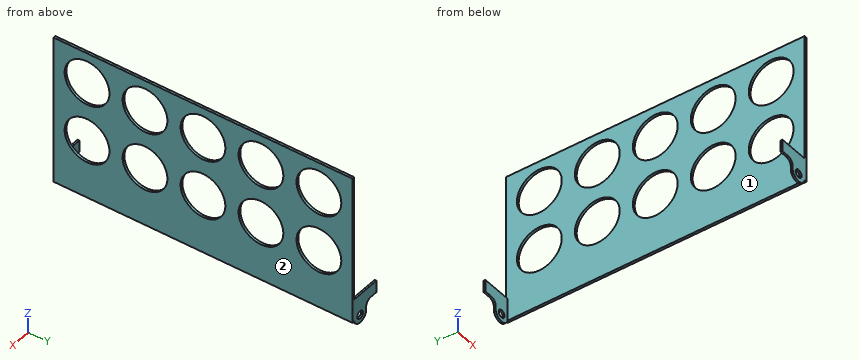
from build123d import *

# Parameters (mm, degrees)
F0_R     = 6.5
F1_DEPTH = 250
F2_W     = 494
F2_H     = 100
F3_DEPTH = 100
F4_R     = 10
F5_W     = 500
F5_H     = 250
F6_DEPTH = 4
F7_R     = 37.5
F8_DEPTH = 25


with BuildPart() as f1:
    # F0 (on Front) → F1 (new body, symmetric)
    with BuildSketch(Plane.XZ):
        with BuildLine():
            Line((-13.5, 15), (-13.5, 0))
            ThreePointArc((-13.5, 0), (-1.356871, -13.431638), (13.227245, -2.7))
            Line((13.227245, -2.7), (13.5, -2.7))
            Line((13.5, -2.7), (13.5, 15))
            Line((13.5, 15), (13.5, 35))
            Line((13.5, 35), (-36.5, 35))
            Line((-36.5, 35), (-36.5, 15))
            Line((-36.5, 15), (-13.5, 15))
        make_face()
        Circle(F0_R, mode=Mode.SUBTRACT)
    extrude(amount=F1_DEPTH, both=True)

    # F2 (on face) → F3 (cut)
    with BuildSketch(Plane.YZ.offset(13.5)):
        Rectangle(F2_W, F2_H)
    extrude(amount=-F3_DEPTH, mode=Mode.SUBTRACT)

    # F4
    f4_edges = [f1.edges().sort_by_distance(p)[0] for p in [
        (-13.5, 248.5, 15),
        (-13.5, -248.5, 15),
    ]]
    fillet(f4_edges, radius=F4_R)

    # F5 (on face) → F6 (join)
    with BuildSketch(Plane.YZ.offset(13.5)):
        with Locations((0, 122.3)):
            Rectangle(F5_W, F5_H)
    extrude(amount=F6_DEPTH)

    # F7 (on face) → F8 (cut)
    with BuildSketch(Plane.YZ.offset(17.5)):
        with Locations((-194, 95.8)):
            Circle(F7_R)
        with Locations((-194, 195.8)):
            Circle(F7_R)
        with Locations((-97, 95.8)):
            Circle(F7_R)
        with Locations((-97, 195.8)):
            Circle(F7_R)
        with Locations((0, 95.8)):
            Circle(F7_R)
        with Locations((0, 195.8)):
            Circle(F7_R)
        with Locations((97, 95.8)):
            Circle(F7_R)
        with Locations((97, 195.8)):
            Circle(F7_R)
        with Locations((194, 95.8)):
            Circle(F7_R)
        with Locations((194, 195.8)):
            Circle(F7_R)
    extrude(amount=-F8_DEPTH, mode=Mode.SUBTRACT)


solid = f1.part
Could you check a few things on this model? Use its own coordinates, in mm. Face numbers are marked on the shaded views. Coordinates: 2 decimals unless noted, no trailing zeros. Loops run counter-clockwise (first coordinate to the right, second up) from the corner with the lowest first, then second, coordinate; pieces in that order, holes last.
1. For P1, Ø3, axis at y = 78, z = 160.5, coming from the -X side; P2, Ø1.5, axis at x = -22.5, y = -248.5, coming from the +Z side; P3, Ø0.9, axis at y = -248.5, z = 1.5, coming from the -X side; P4, Ø21, axis at x = 0, z = 0, coming from the -Y side, each with a flat end and sliding along its axis, tell me the tip position at first contact or that it passes through.
2. We'd pull the mould along Y, two halves only. Please class the marked faces 1 and 2: released by +Y, released by -Y, zero draft, split by the parting line, or undercut.
3. Imagine slicing it at A-A (x = 0). Please give me the cut outline in (y, z), and give its area (3 significant figures).
4. Imagine slicing it at C-C (z = 95.8). Please give me the cut outline in (x, y).
5. Imagine slicing it at B-B (y = 0). Please give me the cut outline in (x, z), and give its area (3 significant figures).
6. I need wall thicknesses on L1, parallel to Z at x = 14.85, y = 0; L2, parallel to Y at x = 16, z = 195; L3, parallel to X at y = 201.5, z = 27. Which ranges of each line are inside material? Lowest first, please.
7. Imagine slicing it at D-D (x = -30). Please give me the cut outline in (y, z), and give its area (3 significant figures).
Computed values:
1. P1: stops at x = 13.5
1. P2: stops at z = 35
1. P3: stops at x = -13.5
1. P4: stops at y = -250
2. face 1: undercut
2. face 2: zero draft
3. outline: (-250, -13.5) - (-247, -13.5) - (-247, -6.5) - (-250, -6.5) - close; (-250, 6.5) - (-247, 6.5) - (-247, 35) - (-250, 35) - close; (247, -13.5) - (250, -13.5) - (250, -6.5) - (247, -6.5) - close; (247, 6.5) - (250, 6.5) - (250, 35) - (247, 35) - close
3. area: 213 mm2
4. outline: (13.5, -250) - (17.5, -250) - (17.5, -231.5) - (13.5, -231.5) - close; (13.5, -156.5) - (17.5, -156.5) - (17.5, -134.5) - (13.5, -134.5) - close; (13.5, -59.5) - (17.5, -59.5) - (17.5, -37.5) - (13.5, -37.5) - close; (13.5, 37.5) - (17.5, 37.5) - (17.5, 59.5) - (13.5, 59.5) - close; (13.5, 134.5) - (17.5, 134.5) - (17.5, 156.5) - (13.5, 156.5) - close; (13.5, 231.5) - (17.5, 231.5) - (17.5, 250) - (13.5, 250) - close
5. outline: (13.5, -2.7) - (17.5, -2.7) - (17.5, 58.3) - (13.5, 58.3) - close; (13.5, 133.3) - (17.5, 133.3) - (17.5, 158.3) - (13.5, 158.3) - close; (13.5, 233.3) - (17.5, 233.3) - (17.5, 247.3) - (13.5, 247.3) - close
5. area: 400 mm2
6. L1: z = -2.7 to 58.3, 133.3 to 158.3, 233.3 to 247.3
6. L2: y = -250 to -231.49, -156.51 to -134.49, -59.51 to -37.49, 37.49 to 59.51, 134.49 to 156.51, 231.49 to 250
6. L3: x = 13.5 to 17.5
7. outline: (-250, 15) - (-247, 15) - (-247, 35) - (-250, 35) - close; (247, 15) - (250, 15) - (250, 35) - (247, 35) - close
7. area: 120 mm2
